Design review of the part built by this model. Coordinates are the model's own, in mm. A direction names the side the tool comes from. Coordinates: 2 decimals unless noted, no trailing zeros. Use a Markdown table: item, result. Add a question column.
Q1. Clearance check with flat-ended pins moving along their axes: pin 1 Ø2 at (y, z) = (-0.5, 221.5) entering from +X; pin 2 Ø6 at (y, z) = (1.5, 100) entering from -X (3 decimals); pin 3 Ø5 at (x, z) = (1, 180.5) entering from -Y (3 decimals). State where each tip first meets the part, or that it passes through.
Q2. Take a section at A-A on z = 145. Count the separate pieces of the cut face and the enclosed holes in it, plus the area to 3 significant figures.
Q3. For faces 1 (the face through (20, 4.186, 148)), 2 (the face through (0, -4.186, 148)), 3 (the face through (10, 8.2, 148)), list the 3-axis set-ups (+Z, -Z, +X, -X, +Y, -Y) from which the entire face can be reached by the end or side of a thin tool; tool diameter is ignored.
Q4. For probe 1 along X at (y, z) = (-8.25, 236) (3 decimals); probe 2 along Y at (x, z) = (20, 172.5); probe 3 along X at (y, z) = (-6.5, 241.5), list the stretches that pass through material, from the lowest coordinate up.
Q5. Draft analysis for pull direction Y (two halves, no side actions). For faces 4 (the face through (15.814, 0, 148)), 5 (the face through (5, 5, 300)), 6 (the face through (0, 4.186, 148)), state which applies: pulls with the +Y half, pulls with the -Y half, needs draft (parallel to the pull), parting line crosses it, or undercut.
Autodesk Inventor part; units mm, degrees
ref_plane "Płaszczyzna konstrukcyjna1" through (10, 8.2, 0) normal (1, 0, 0) x (0, 0, -1)
ref_plane "YZ Plane" through (0, 0, 0) normal (1, 0, 0) x (0, 1, 0)
ref_plane "XZ Plane" through (0, 0, 0) normal (0, 1, 0) x (-1, 0, 0)
sketch "Szkic1" plane through (0, 0, 0) normal (0, 0, 1) x (1, 0, 0)
  circle A0 centre (0, 0) radius 2.1
  line L0 (-10, 10) -> (10, 10)
  line L1 (10, 10) -> (10, -10)
  line L2 (10, -10) -> (-10, -10)
  line L3 (-10, -10) -> (-10, 10)
  line L4 (-10, -10) -> (10, 10) construction
  line L5 (10, -10) -> (-10, 10) construction
  line L6 (-10, 8.2) -> (10, 8.2)
  line L7 (-10, -8.2) -> (10, -8.2)
  line L8 (-8.2, 10) -> (-8.2, -10)
  line L9 (10, 10) -> (30, 10)
  line L10 (30, 10) -> (30, -10)
  line L11 (30, -10) -> (10, -10)
  line L12 (10, -10) -> (10, 10)
  line L13 (-4.1857, -4.1857) -> (4.1857, -4.1857)
  line L14 (4.1857, -4.1857) -> (4.1857, 4.1857)
  line L15 (4.1857, 4.1857) -> (-4.1857, 4.1857)
  line L16 (-4.1857, 4.1857) -> (-4.1857, -4.1857)
  line L17 (-8.2, 7.1393) -> (-4.1857, 3.125)
  line L18 (-7.1393, 8.2) -> (-3.125, 4.1857)
  line L19 (-4.925, 10) -> (-3.125, 8.2)
  line L20 (4.925, 10) -> (3.125, 8.2)
  line L21 (-3.125, -8.2) -> (-4.925, -10)
  line L22 (3.125, -8.2) -> (4.925, -10)
  line L23 (-8.2, -7.1393) -> (-4.1857, -3.125)
  line L24 (-7.1393, -8.2) -> (-3.125, -4.1857)
  line L25 (3.125, -4.1857) -> (7.1393, -8.2)
  line L26 (4.1857, -3.125) -> (7.3007, -6.24)
  line L27 (4.1857, 3.125) -> (7.3007, 6.24)
  line L28 (3.125, 4.1857) -> (7.1393, 8.2)
  line L29 (-5.4993, 8.2) -> (-5.4993, 6.56)
  line L30 (5.4993, 8.2) -> (5.4993, 6.56)
  line L31 (-8.2, 5.4993) -> (-6.56, 5.4993)
  line L32 (-8.2, -5.4993) -> (-6.56, -5.4993)
  line L33 (-5.4993, -6.56) -> (-5.4993, -8.2)
  line L34 (5.4993, -6.56) -> (5.4993, -8.2)
  line L35 (-8.2, 3.125) -> (-10, 4.925)
  line L36 (-8.2, -3.125) -> (-10, -4.925)
  line L37 (7.3007, 6.24) -> (7.3007, 8.2)
  line L38 (7.3007, -6.24) -> (7.3007, -8.2)
  point P0 (0, -8.2)
  point P1 (-8.2, -8.2)
  point P2 (-8.2, 8.2)
  dimension "d0" = 4.2
  dimension "d1" = 20
  dimension "d2" = 1.8
  dimension "d4" = 20
  dimension "d5" = 20
  dimension "d6" = 1.8
  dimension "d7" = 1.8
  dimension "d8" = 1.5
  dimension "d9" = 0.75
  dimension "d10" = 135
  dimension "d11" = 6.25
  dimension "d12" = 3.125
  dimension "d13" = 1.5
  dimension "d14" = 1.5
  dimension "d15" = 1.5
  dimension "d16" = 0.75
  dimension "d17" = 0.75
  dimension "d18" = 0.75
  dimension "d19" = 1.64
  dimension "d20" = 1.64
  dimension "d21" = 1.64
  dimension "d22" = 1.64
  dimension "d23" = 1.64
  dimension "d24" = 1.64
  dimension "d25" = 45
  dimension "d30" = 1.96
  dimension "d31" = 1.96
extrude "Wyciągnięcie proste1" add sketch "Szkic1" along normal blind 300 contours L0 L8 L6 L3 | L0 L19 L6 L8 | L6 L8 L35 L3 | L6 L18 L15 L16 L17 L8 | L0 L1 L6 L20 | L6 L29 L18 | L17 L31 L8 | L36 L8 L7 L3 | L7 L8 L2 L3 | L6 L28 L30 | L15 L14 L13 L16 | L8 L23 L16 L13 L24 L7 | L7 L21 L2 L8 | L32 L23 L8 | L1 L2 L22 L7 | L37 L27 L14 L15 L28 L6 | L24 L33 L7 | L7 L25 L13 L14 L26 L38 | L7 L34 L25
ref_plane "Płaszczyzna konstrukcyjna1" through (10, 8.2, 0) normal (1, 0, 0) x (0, 0, -1)
mirror "Odbij1" about plane through (10, 8.2, 0) normal (1, 0, 0) of "Wyciągnięcie proste1"
fillet "Zaokrąglenie1" radius 0.5 4 edges at (-10, 10, 150) (-10, -10, 150) (30, 10, 150) (30, -10, 150)
properties part number "2040vslot_long"
Answer list:
| question | item | result |
|---|---|---|
| 1 | pin 1 | x = 24.19 |
| 1 | pin 2 | x = -9.575 |
| 1 | pin 3 | y = -8.575 |
| 2 | separate pieces | 1 |
| 2 | enclosed holes | 3 |
| 2 | area | 307 mm² |
| 3 | face 1 | +Z, -Z, +Y |
| 3 | face 2 | +Z, -Z, -Y |
| 3 | face 3 | +Z, -Z |
| 4 | probe 1 | -10 to -3.175, 3.175 to 16.825, 23.175 to 30 |
| 4 | probe 2 | -4.19 to -2.1, 2.1 to 4.19 |
| 4 | probe 3 | -10 to -5.44, 5.44 to 7.3, 12.7 to 14.56, 25.44 to 30 |
| 5 | face 4 | undercut |
| 5 | face 5 | needs draft |
| 5 | face 6 | pulls with the +Y half |
